from build123d import *

# Parameters (mm, degrees)
BOSS_EXTRUDE1_DEPTH      = 2
BOSS_EXTRUDE1_DEPTH_BACK = 4
BOSS_EXTRUDE2_DEPTH      = 2
BOSS_EXTRUDE3_DEPTH      = 2


with BuildPart() as part:
    # Sketch1 → Boss-Extrude1 (new, two sides: drawn at the far end of the back side and taken through both)
    with BuildSketch(Plane(origin=(0, 0, 0), x_dir=(0, 0, -1), z_dir=(1, 0, 0)).offset(-BOSS_EXTRUDE1_DEPTH_BACK)):
        with BuildLine():
            Line((-5.5, 0), (-3.5, 0))
            ThreePointArc((-3.5, 0), (0, 3.5), (3.5, 0))
            ThreePointArc((3.5, 0), (3.446827136, -0.607768622), (3.288924173, -1.197070502))
            Line((3.288924173, -1.197070502), (5.168309414, -1.881110788))
            ThreePointArc((5.168309414, -1.881110788), (5.416442642, -0.955064977), (5.5, 0))
            ThreePointArc((5.5, 0), (0, 5.5), (-5.5, 0))
        make_face()
        with BuildLine():
            Line((5.168309414, -1.881110788), (3.288924173, -1.197070502))
            ThreePointArc((3.288924173, -1.197070502), (3.88659665, -2.478783266), (5.168309414, -1.881110788))
        make_face()
        with BuildLine():
            ThreePointArc((-3.288924173, -1.197070502), (-3.446827136, -0.607768622), (-3.5, 0))
            Line((-3.5, 0), (-5.5, 0))
            ThreePointArc((-5.5, 0), (-5.416442642, -0.955064977), (-5.168309414, -1.881110788))
            Line((-5.168309414, -1.881110788), (-4.228616794, -1.539090645))
            Line((-4.228616794, -1.539090645), (-3.288924173, -1.197070502))
        make_face()
        with BuildLine():
            ThreePointArc((-5.168309414, -1.881110788), (-3.88659665, -2.478783266), (-3.288924173, -1.197070502))
            Line((-3.288924173, -1.197070502), (-4.228616794, -1.539090645))
            Line((-4.228616794, -1.539090645), (-5.168309414, -1.881110788))
        make_face()
    extrude(amount=BOSS_EXTRUDE1_DEPTH + BOSS_EXTRUDE1_DEPTH_BACK)

    # Sketch2 → Boss-Extrude2 (add)
    with BuildSketch(Plane(origin=(0, 0, 0), x_dir=(0, 0, -1), z_dir=(1, 0, 0))):
        Polygon((-2, 3.5), (0, 3.5), (2, 3.5), (2, 55.5), (-2, 55.5), align=None)
    extrude(amount=BOSS_EXTRUDE2_DEPTH)

    # Sketch3 → Boss-Extrude3 (add)
    with BuildSketch(Plane(origin=(0, 0, 0), x_dir=(0, 0, -1), z_dir=(1, 0, 0))):
        Polygon((1, 55.5), (0, 55.5), (-1, 55.5), (-1, 3.5), (1, 3.5), align=None)
    extrude(amount=-BOSS_EXTRUDE3_DEPTH)


solid = part.part
Geometry check sheet. Reference: the model listing, model coordinates, mm. A direction names the side the tool comes from. Round coordinates to 2 decimals unless told otherwise and drop trailing zeros. Order: outer loops, then holes, each group sorted by start corner. A loop starts at its lowest first (then second) coordinate and runs counter-clockwise, first axis right, second up. Notation, with made-up numbers: M 8,21.5 L 30,21.5 A17 ccw 30,30.5 Z; hole C 89,-18.75 d5. An arc over 180 degrees is marked long. Answer in a Markdown table with one row per item. Add a question column.
Item 1: Material ranges on L1, parallel to X at y = 22, z = 0.25; L2, parallel to Y at x = -0.6, z = 0.25, recorded low to high. Write a range as [from, to].
Item 2: Depth check by flat-ended pin: pin 1 Ø1.6 at (x, y) = (1, 29.5) entering from -Z; pin 2 Ø0.6 at (y, z) = (18.5, 0.5) entering from -X; pin 3 Ø0.8 at (y, z) = (30, -1.5) entering from -X. Enter the tip coordinate at first touch or a pass-through.
Item 3: Sectioned sample at B-B, the plane y = 29.5. Enter the section's corners in (x, z).
Item 4: Draft check along Z on faces 6 (the face through (-1, 30, -1)), 7 (the face through (-4, 4, 0)), 8 (the face through (-1.042, -2.486, 3.907)). Enter one of: released by +Z, released by -Z, zero draft, split by the parting line, or undercut.
Item 5: Sectioned sample at A-A, the plane x = -0.95. Enter the section's corners in (y, z), plus the area to 3 significant figures.
Item 6: Sectioned sample at C-C, the plane y = 2. Enter the section's corners in (x, z), plus the area to 3 significant figures.
Item 7: Set-up check for faces 1 (the face through (0, 30.7, 1.5)), 2 (the face through (-2, 31, 0)), 3 (the face through (0, 30.7, -1.5)), 4 (the face through (1, 31, 2)), 5 (the face through (1, 30, -2)): record each of +Z, -Z, +X, -X, +Y, -Y from which the full face is reachable in a straight line by a thin tool's end or side.
Item 8: Sectioned sample at D-D, the plane z = 0. Enter the section's corners in (x, y), plus the area to 3 significant figures.
Filled in:
| question | item | result |
|---|---|---|
| 1 | L1 | x = [-2, 2] |
| 1 | L2 | y = [3.49, 55.5] |
| 2 | pin 1 | stops at z = -2 |
| 2 | pin 2 | stops at x = -2 |
| 2 | pin 3 | stops at x = 0 |
| 3 | outline | M -2,-1 L 0,-1 L 0,-2 L 2,-2 L 2,2 L 0,2 L 0,1 L -2,1 Z |
| 4 | face 6 | released by -Z |
| 4 | face 7 | zero draft |
| 4 | face 8 | undercut |
| 5 | outline | M -1.88,-5.17 A5.5 ccw 5.41,-1 L 55.5,-1 L 55.5,1 L 5.41,1 A5.5 ccw -1.88,5.17 A1 ccw -1.2,3.29 A3.5 cw long -1.2,-3.29 A1 ccw Z |
| 5 | area | 138 mm² |
| 6 | outline | M -4,-5.12 L 2,-5.12 L 2,-2.87 L -4,-2.87 Z; M -4,2.87 L 2,2.87 L 2,5.12 L -4,5.12 Z |
| 6 | area | 27.0 mm² |
| 7 | face 1 | +Z, -X, +Y |
| 7 | face 2 | +Z, -Z, -X, +Y |
| 7 | face 3 | -Z, -X, +Y |
| 7 | face 4 | +Z, +X, -X, +Y |
| 7 | face 5 | -Z, +X, -X, +Y |
| 8 | outline | M -4,3.5 L 2,3.5 L 2,55.5 L -2,55.5 L -2,5.5 L -4,5.5 Z |
| 8 | area | 212 mm² |
